Geometry: final body of the model. Coordinates: model frame, mm. A direction names the side the tool comes from. Give positions to 0.01 mm unless a question says otherwise; leave off trailing zeros. Order: outer loops, then holes, each group sorted by start corner. A loop starts at its lowest first (then second) coordinate and runs counter-clockwise, first axis right, second up. Notation, with made-up numbers: (-11.75, -35.5) -> (12.25, -35.5) arc R19 ccw to (12.25, 0.5) -> close; hole circle Ø3 at (54, -14). An arc over 180 degrees is marked (long way). Write item = value, one per line.
```python
from build123d import *

# Parameters (mm, degrees)
PCB_DIMENSIONS_W    = 47.716732244
PCB_DIMENSIONS_H    = 77.636732244
BOSS_EXTRUDE3_DEPTH = 1.5
SKETCH5_W           = 43.474091557
SKETCH5_H           = 73.394091557
SKETCH5_W_2         = 39.23145087
SKETCH5_H_2         = 69.15145087
BOSS_EXTRUDE4_DEPTH = 1.8
FILLET1_R           = 1
SKETCH6_W           = 12
SKETCH6_H           = 31.966906412
SKETCH6_H_2         = 32.033093588
BOSS_EXTRUDE5_DEPTH = 10
SKETCH7_W           = 48
SKETCH7_H           = 6
CUT_EXTRUDE1_DEPTH  = 24
FILLET2_R           = 6
FILLET3_R           = 1
SCALE1_SCALE        = 0.99


with BuildPart() as part:
    # PCB Dimensions → Boss-Extrude3 (new body)
    with BuildSketch(Plane(origin=(0, 0, 0), x_dir=(1, 0, 0), z_dir=(0, 1, 0))):
        with Locations((20.322832216, -35.282832216)):
            Rectangle(PCB_DIMENSIONS_W, PCB_DIMENSIONS_H)
    extrude(amount=BOSS_EXTRUDE3_DEPTH)

    # Sketch5 → Boss-Extrude4 (add)
    with BuildSketch(Plane(origin=(0, 1.5, 0), x_dir=(1, 0, 0), z_dir=(0, 1, 0))):
        with Locations((20.322832217, -35.282832217)):
            Rectangle(SKETCH5_W, SKETCH5_H)
        with Locations((20.322832216, -35.282832216)):
            Rectangle(SKETCH5_W_2, SKETCH5_H_2, mode=Mode.SUBTRACT)
    extrude(amount=BOSS_EXTRUDE4_DEPTH)

    # Fillet1
    fillet1_edges = [part.edges().sort_by_distance(p)[0] for p in [
        (-1.414213562, 2.4, -1.414213562),
        (-1.414213562, 2.4, 71.979877995),
        (42.059877995, 2.4, 71.979877995),
        (42.059877995, 2.4, -1.414213562),
        (0.707106781, 2.4, 0.707106781),
        (0.707106781, 2.4, 69.858557651),
        (39.938557651, 2.4, 69.858557651),
        (39.938557651, 2.4, 0.707106781),
    ]]
    fillet(fillet1_edges, radius=FILLET1_R)

    # Sketch6 → Boss-Extrude5 (add)
    with BuildSketch(Plane.XZ):
        with Locations((14.322832216, 51.266285422)):
            Rectangle(SKETCH6_W, SKETCH6_H)
        with Locations((26.322832216, 51.266285422)):
            Rectangle(SKETCH6_W, SKETCH6_H)
        with Locations((14.322832216, 19.266285422)):
            Rectangle(SKETCH6_W, SKETCH6_H_2)
        with Locations((26.322832216, 19.266285422)):
            Rectangle(SKETCH6_W, SKETCH6_H_2)
    extrude(amount=BOSS_EXTRUDE5_DEPTH)

    # Sketch7 → Cut-Extrude1 (cut)
    with BuildSketch(Plane(origin=(32.322832216, 0, 0), x_dir=(0, 0, -1), z_dir=(1, 0, 0))):
        with Locations((-35.249738628, -3)):
            Rectangle(SKETCH7_W, SKETCH7_H)
    extrude(amount=-CUT_EXTRUDE1_DEPTH, mode=Mode.SUBTRACT)

    # Fillet2
    fillet2_edges = [part.edges().sort_by_distance(p)[0] for p in [
        (20.322832216, -10, 67.249738628),
        (20.322832216, -10, 3.249738628),
    ]]
    fillet(fillet2_edges, radius=FILLET2_R)

    # Fillet3
    fillet3_edges = [part.edges().sort_by_distance(p)[0] for p in [
        (20.322832216, -6, 59.249738628),
        (20.322832216, -6, 11.249738628),
    ]]
    fillet(fillet3_edges, radius=FILLET3_R)


with BuildPart() as part_1:
    # Scale1: scaled about (20.322832216, -3.218350849, 35.264379677)
    add(part.part.scale(SCALE1_SCALE).moved(Location((0.203228322, -0.032183508, 0.352643797))))


solid = part_1.part
```
1) Line query: line 1 (Z direction, x = 25, y = 2); line 2 (Z direction, x = 24, y = -3); line 3 (Y direction, x = 28, z = 32). Output: solid intervals per line, ascending. Write a range as from..to.
Check sheet entries:
line_1 = -1.05..1.05, 69.51..71.61
line_2 = 3.57..11.49, 59.01..66.93
line_3 = -9.93..-5.97, -0.03..1.45
2) Section query B-B (z = 42). Output: boundary loops of the cut face in (x, y).
Check sheet entries:
outline = (-3.3, -0.03) -> (43.94, -0.03) -> (43.94, 1.45) -> (41.84, 1.45) -> (41.84, 3.23) -> (39.74, 3.23) -> (39.74, 1.45) -> (0.9, 1.45) -> (0.9, 3.23) -> (-1.2, 3.23) -> (-1.2, 1.45) -> (-3.3, 1.45) -> close; (8.44, -9.93) -> (32.2, -9.93) -> (32.2, -5.97) -> (8.44, -5.97) -> close
3) Section query C-C (y = -2.25). Output: boundary loops of the cut face in (x, z), plus the area to 3 significant figures.
Check sheet entries:
outline = (8.44, 3.57) -> (32.2, 3.57) -> (32.2, 11.49) -> (8.44, 11.49) -> close; (8.44, 59.01) -> (32.2, 59.01) -> (32.2, 66.93) -> (8.44, 66.93) -> close
area = 376 mm²
4) First-contact query: P1, Ø5, axis at x = 39, z = 52.5, coming from the +Y side; P2, Ø4, axis at x = 28, z = 35.5, coming from the +Y side; P3, Ø2, axis at y = 2.5, z = 25, coming from the +X side; P4, Ø1.2, axis at x = 20, y = -2.5, coming from the +Z side. Flat tips, straight axial feed; report the tip coordinate or a pass-through.
Check sheet entries:
P1 = 3.23
P2 = 1.45
P3 = 41.84
P4 = 66.93
5) Section query A-A (y = 2.25). Output: boundary loops of the cut face in (x, z).
Check sheet entries:
outline = (-1.2, -0.06) arc R0.99 ccw to (-0.21, -1.05) -> (40.85, -1.05) arc R0.99 ccw to (41.84, -0.06) -> (41.84, 70.62) arc R0.99 ccw to (40.85, 71.61) -> (-0.21, 71.61) arc R0.99 ccw to (-1.2, 70.62) -> close; hole (0.9, 2.04) arc R0.99 ccw to (1.89, 1.05) -> (38.75, 1.05) arc R0.99 ccw to (39.74, 2.04) -> (39.74, 68.52) arc R0.99 ccw to (38.75, 69.51) -> (1.89, 69.51) arc R0.99 ccw to (0.9, 68.52) -> close
6) Reachability of faces 4 (the face through (41.843, 2, 36)), 5 (the face through (20, 2, 69.513)), 6 (the face through (20, -5.972, 36)), 7 (the face through (20, -2, 3.57)), 8 (the face through (20, 2, -1.047)) from +Z, -Z, +X, -X, +Y, -Y: full face, straight path, thin tool, end or side. Return the list, or none.
Check sheet entries:
face_4 = +Z, -Z, +X, +Y
face_5 = +Y
face_6 = +X, -X
face_7 = -Z, +X, -X, -Y
face_8 = -Z, +X, -X, +Y
7) Section query D-D (x = 31). Output: boundary loops of the cut face in (y, z), plus the area to 3 significant figures.
Check sheet entries:
outline = (-9.93, 9.51) arc R5.94 ccw to (-3.99, 3.57) -> (-0.03, 3.57) -> (-0.03, -3.15) -> (1.45, -3.15) -> (1.45, -1.05) -> (3.23, -1.05) -> (3.23, 1.05) -> (1.45, 1.05) -> (1.45, 69.51) -> (3.23, 69.51) -> (3.23, 71.61) -> (1.45, 71.61) -> (1.45, 73.71) -> (-0.03, 73.71) -> (-0.03, 66.93) -> (-3.99, 66.93) arc R5.94 ccw to (-9.93, 60.99) -> close; hole (-5.97, 12.48) arc R0.99 ccw to (-4.98, 11.49) -> (-0.03, 11.49) -> (-0.03, 59.01) -> (-4.98, 59.01) arc R0.99 ccw to (-5.97, 58.02) -> close
area = 452 mm²
8) Mould query, pull axis Y, two halves, no side actions, for faces 1 (the face through (39.742, 2, 36)), 2 (the face through (20, 1.453, 35)), 3 (the face through (20, -0.032, 35)). Classes: +Y half, -Y half, draft (parallel to the pull), parting line (faces both ways), or undercut.
Check sheet entries:
face_1 = draft
face_2 = +Y half
face_3 = undercut
